Verification items for the finished model (mm, model axes). Round coordinates to 2 decimals unless told otherwise and drop trailing zeros. Order: outer loops, then holes, each group sorted by start corner. A loop starts at its lowest first (then second) coordinate and runs counter-clockwise, first axis right, second up. Notation, with made-up numbers: M 14,62 L 38,62 A12 ccw 38,69 Z; hole C -26.75,-38 d8. An arc over 180 degrees is marked long. Return JSON: item names as keys, results as strings. Group by question number.
from build123d import *

# Parameters (mm, degrees)
BOSS_EXTRUDE1_DEPTH = 5
CUT_EXTRUDE1_REACH  = 75.47
SKETCH2_W           = 2.306675789
SKETCH2_H           = 6.75004694
CUT_EXTRUDE2_REACH  = 75.371
SKETCH3_W           = 101.6
SKETCH3_H           = 1.753256074


with BuildPart() as part:
    # Sketch1 → Boss-Extrude1 (new, symmetric)
    with BuildSketch(Plane(origin=(0, 0, 0), x_dir=(1, 0, 0), z_dir=(0, 1, 0))):
        Polygon((-73.023921726, 9.380838376), (-66.673921726, 9.380838376), (-66.673921726, 4.300838376), (34.926078274, 4.300838376), (34.926078274, 3.030838376), (-66.673921726, 3.030838376), (-73.023921726, 3.030838376), align=None)
    extrude(amount=BOSS_EXTRUDE1_DEPTH, both=True)

    # Sketch2 → Cut-Extrude1 (cut, up to next)
    with BuildSketch(Plane(origin=(0, 0, -9.380838376), x_dir=(-1, 0, 0), z_dir=(0, 0, -1)), mode=Mode.PRIVATE) as cut_extrude1_sk1:
        with Locations((70.270606821, -0.140509405)):
            Rectangle(SKETCH2_W, SKETCH2_H)
    cut_extrude1_tool1 = extrude(cut_extrude1_sk1.sketch, amount=-CUT_EXTRUDE1_REACH, mode=Mode.PRIVATE) & part.part
    add(cut_extrude1_tool1.solids().sort_by_distance((-70.270607, -0.140509, -9.380838))[0], mode=Mode.SUBTRACT)

    # Sketch3 → Cut-Extrude2 (cut, up to next)
    with BuildSketch(Plane(origin=(0, 0, -4.300838376), x_dir=(-1, 0, 0), z_dir=(0, 0, -1)), mode=Mode.PRIVATE) as cut_extrude2_sk1:
        with Locations((15.873921726, 4.123371963)):
            Rectangle(SKETCH3_W, SKETCH3_H)
    cut_extrude2_tool1 = extrude(cut_extrude2_sk1.sketch, amount=-CUT_EXTRUDE2_REACH, mode=Mode.PRIVATE) & part.part
    # Sketch3 → Cut-Extrude2 (cut, up to next)
    with BuildSketch(Plane(origin=(0, 0, -4.300838376), x_dir=(-1, 0, 0), z_dir=(0, 0, -1)), mode=Mode.PRIVATE) as cut_extrude2_sk2:
        with Locations((15.873921726, -4.123371963)):
            Rectangle(SKETCH3_W, SKETCH3_H)
    cut_extrude2_tool2 = extrude(cut_extrude2_sk2.sketch, amount=-CUT_EXTRUDE2_REACH, mode=Mode.PRIVATE) & part.part
    add(cut_extrude2_tool1.solids().sort_by_distance((-15.873922, 4.123372, -4.300838))[0], mode=Mode.SUBTRACT)
    add(cut_extrude2_tool2.solids().sort_by_distance((-15.873922, -4.123372, -4.300838))[0], mode=Mode.SUBTRACT)


solid = part.part
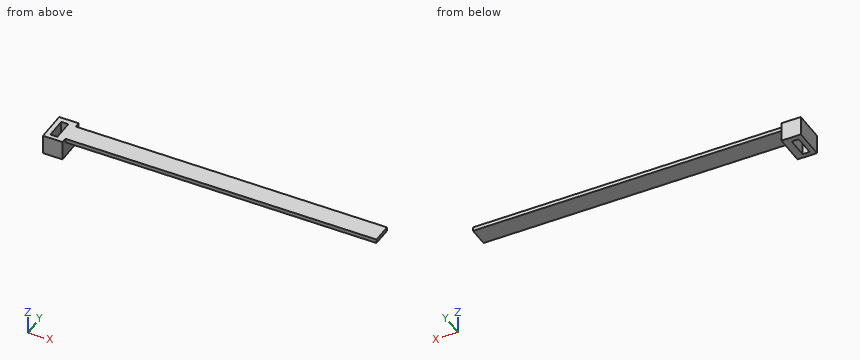
1. Cross-section at A-A (y = -1). Enter the section's corners in (x, z).
2. Cross-section at C-C (x = -17). Enter the section's corners in (y, z), plus the area to 3 significant figures.
3. Go/stop test with flat-tipped pins: pin 1 (6 mm diameter, centred on x = 9, y = -3, fed in from -Z); pin 2 (3 mm diameter, centred on x = -35, z = -4.5, fed in from -Y); pin 3 (2 mm diameter, centred on x = 8.5, z = -4.5, fed in from +Y). Record where each tip stops, or that it passes through.
4. Thickness scan on line 1 along X through (y, z) = (1.75, -7.25); line 2 along X through (y, z) = (3, -4.25); line 3 along Z through (x, y) = (-12.5, -2). Record the ranges inside material, lowest first. Write a range as from..to.
5. Cross-section at B-B (z = -8.25). Enter the section's corners in (x, y).
Computed:
{
 "1": {"outline": "M -73.02,-9.38 L -71.42,-9.38 L -71.42,-3.03 L -73.02,-3.03 Z; M -69.12,-9.38 L -66.67,-9.38 L -66.67,-4.3 L 34.93,-4.3 L 34.93,-3.03 L -69.12,-3.03 Z"},
 "2": {"outline": "M -3.25,-4.3 L 3.25,-4.3 L 3.25,-3.03 L -3.25,-3.03 Z", "area": "8.25 mm²"},
 "3": {"pin 1": "stops at z = -4.3", "pin 2": "stops at y = -3.25", "pin 3": "stops at y = 3.25"},
 "4": {"line 1": "x = -73.02..-71.42, -69.12..-66.67", "line 2": "x = -73.02..-71.42, -69.12..34.93", "line 3": "z = -4.3..-3.03"},
 "5": {"outline": "M -73.02,-5 L -66.67,-5 L -66.67,5 L -73.02,5 Z; hole M -71.42,-3.52 L -69.12,-3.52 L -69.12,3.23 L -71.42,3.23 Z"}
}
